Part print with two shaded views. Sizes in mm from the minimum x, y, z corner. A direction names the side the tool comes from. Round coordinates to 2 decimals unless told otherwise and drop trailing zeros. Write each loop counter-clockwise with the first axis right and the second up, starting at its lowest first coordinate (ties: lowest second). Pieces come first, ordered by that corner, then holes. Notation, with made-up numbers: (5.25, 12) -> (58.25, 12) arc R31 cw to (58.25, 45) -> close; hole circle Ø11 at (39, 34). An arc over 180 degrees is marked (long way). Return JSON: item names as keys, results as strings.
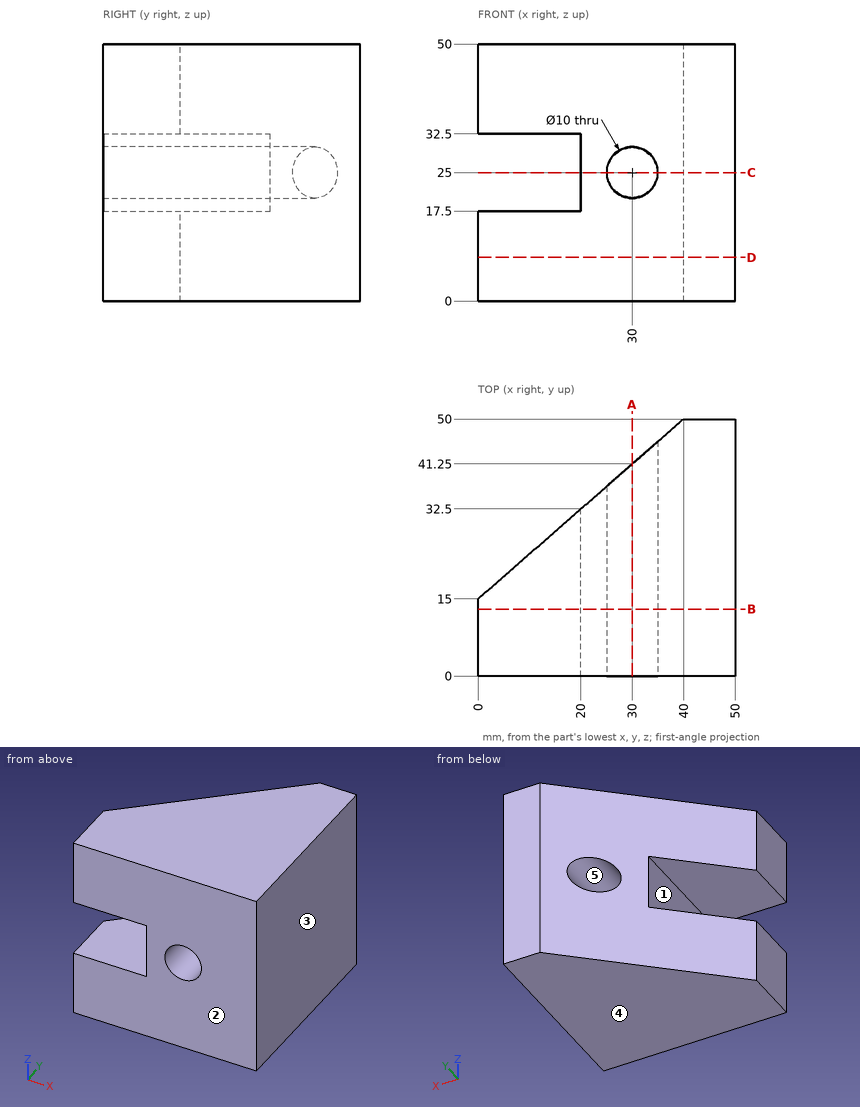
Q1. Saw through at D-D on z = 8.5. List the corners of the cut face in (x, y), then the cut area to 3 significant figures.
Verdict:
{"outline": "(0, 0) -> (50, 0) -> (50, 50) -> (40, 50) -> (0, 15) -> close", "area": "1,800 mm²"}
Q2. 3-axis set-ups, long thin cutter, end or side, ignore diameter. For the marked faces 1 and 2: which of +Z, -Z, +X, -X, +Y, -Y reach the whole face in a straight line?
Verdict:
{"face 1": "-X, +Y, -Y", "face 2": "+Z, -Z, +X, -X, -Y"}
Q3. Two-plate mould, pull along Z, no slides. Class the marked faces 3, 4 and 5: +Z half, -Z half, draft (parallel to the pull), parting line (faces both ways), or undercut.
Verdict:
{"face 3": "draft", "face 4": "-Z half", "face 5": "undercut"}
Q4. Wall check: L1, parallel to Z at x = 14, y = 9.5; L2, parallel to X at y = 25.5, z = 25; L3, parallel to Z at x = 30, y = 18. Give the ranges that are in metal, low to high.
Verdict:
{"L1": "z = 0 to 17.5, 32.5 to 50", "L2": "x = 20 to 25, 35 to 50", "L3": "z = 0 to 20, 30 to 50"}
Q5. Saw through at A-A on x = 30. List the corners of the cut face in (y, z).
Verdict:
{"outline": "(0, 0) -> (41.25, 0) -> (41.25, 20) -> (0, 20) -> close; (0, 30) -> (41.25, 30) -> (41.25, 50) -> (0, 50) -> close"}
Q6. Saw through at C-C on z = 25. List the corners of the cut face in (x, y) (3 decimals).
Verdict:
{"outline": "(20, 0) -> (25, 0) -> (25, 36.875) -> (20, 32.5) -> close; (35, 0) -> (50, 0) -> (50, 50) -> (40, 50) -> (35, 45.625) -> close"}
Q7. Pin check, flat tips, straight feed: pin 1 Ø3 at (x, z) = (7, 7.5) entering from +Y; pin 2 Ø4.5 at (y, z) = (21.5, 27) entering from -X. Stop position of each tip, or through.
Verdict:
{"pin 1": "stops at y = 22.44", "pin 2": "stops at x = 20"}
Q8. Saw through at B-B on y = 13. List the corners of the cut face in (x, z).
Verdict:
{"outline": "(0, 0) -> (50, 0) -> (50, 50) -> (0, 50) -> (0, 32.5) -> (20, 32.5) -> (20, 17.5) -> (0, 17.5) -> close; hole circle Ø10 at (30, 25)"}
